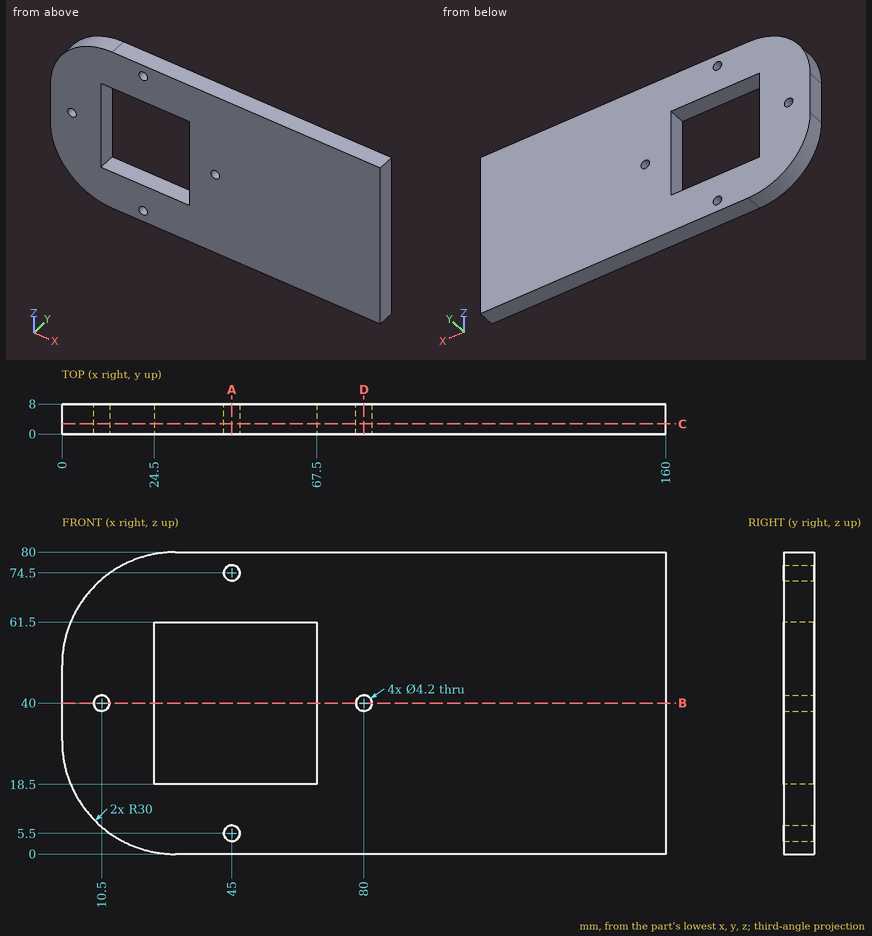
Design review of the part shown in the three views and the two pictorial views. Dimensions are in mm from the part's minimum x, y and z. Round coordinates to 2 decimals unless told otherwise and drop trailing zeros. Loops run counter-clockwise (first coordinate to the right, second up) from the corner with the lowest first, then second, coordinate; pieces in that order, holes last. Notation, with made-up numbers: (25.5, 10.25) - (81.5, 10.25) arc R19 cw to (81.5, 35.25) - close; hole circle Ø8 at (66.5, -2.75). An arc over 180 degrees is marked (long way). Answer as CSV lines item,"result".
(1) Consider section A-A on x = 45. Give the boundary of the cut face in (y, z), then the cut area to 3 significant figures.
Checked values:
outline,"(0, 0) - (8, 0) - (8, 3.4) - (0, 3.4) - close; (0, 7.6) - (8, 7.6) - (8, 18.5) - (0, 18.5) - close; (0, 61.5) - (8, 61.5) - (8, 72.4) - (0, 72.4) - close; (0, 76.6) - (8, 76.6) - (8, 80) - (0, 80) - close"
area,"229 mm2"
(2) Consider section D-D on x = 80. Give the boundary of the cut face in (y, z), then the cut area to 3 significant figures.
Checked values:
outline,"(0, 0) - (8, 0) - (8, 37.9) - (0, 37.9) - close; (0, 42.1) - (8, 42.1) - (8, 80) - (0, 80) - close"
area,"606 mm2"
(3) Insertion check: P1, Ø3.5, axis at x = 80, z = 40, coming from the -Y side; P2, Ø4, axis at x = 17.5, y = 1.5, coming from the +Z side; P3, Ø1.5, axis at y = 1, z = 10, coming from the -X side. Each pin has a flat end and moves straight along its axis. Give the tip position at first contact, or say it passes through.
Checked values:
P1,"passes through"
P2,"stops at z = 78.1"
P3,"stops at x = 6.99"
(4) Consider section C-C on y = 2.75. Give the boundary of the cut face in (x, z), then the cut area to 3 significant figures.
Checked values:
outline,"(0, 30) arc R30 ccw to (30, 0) - (160, 0) - (160, 80) - (30, 80) arc R30 ccw to (0, 50) - close; hole circle Ø4.2 at (10.5, 40); hole (24.5, 18.5) - (67.5, 18.5) - (67.5, 61.5) - (24.5, 61.5) - close; hole circle Ø4.2 at (45, 5.5); hole circle Ø4.2 at (45, 74.5); hole circle Ø4.2 at (80, 40)"
area,"10,500 mm2"
(5) Consider section B-B on z = 40. Give the boundary of the cut face in (x, y).
Checked values:
outline,"(0, 0) - (8.4, 0) - (8.4, 8) - (0, 8) - close; (12.6, 0) - (24.5, 0) - (24.5, 8) - (12.6, 8) - close; (67.5, 0) - (77.9, 0) - (77.9, 8) - (67.5, 8) - close; (82.1, 0) - (160, 0) - (160, 8) - (82.1, 8) - close"
(6) Wall thickness on line 1 (Z direction, x = 45, y = 6.5); line 2 (X direction, y = 4, z = 40); line 3 (X direction, y = 0.5, z = 44.5): over which ranges is each line inside the solid? List them lowest first.
Checked values:
line 1,"z = 0 to 3.4, 7.6 to 18.5, 61.5 to 72.4, 76.6 to 80"
line 2,"x = 0 to 8.4, 12.6 to 24.5, 67.5 to 77.9, 82.1 to 160"
line 3,"x = 0 to 24.5, 67.5 to 160"
